Read the model definition and answer for the solid it produces. Units are mm, in the model's axes. Face numbers are marked on the shaded views. A direction names the side the tool comes from. Coordinates: 2 decimals unless noted, no trailing zeros. Write each loop counter-clockwise with the first axis right and the second up, starting at its lowest first coordinate (ties: lowest second). Pieces come first, ordered by that corner, then holes. Notation, with made-up numbers: (10.25, 60) -> (68.25, 60) arc R23 ccw to (68.25, 97) -> close; hole circle Ø11 at (-22, -4). An arc over 180 degrees is marked (long way). Answer as a JSON object with one key per item and string values. Group by question number.
(1) Find section C-C (z = -11). Give the vertices of the cut face in (x, y).
(2) Find section D-D (y = 47). Count the separate pieces of the cut face and the enclosed holes in it, then the cut area to 3 significant figures.
(3) Find section B-B (y = 22). Give the vertices of the cut face in (x, z) (3 decimals).
(4) Which of the six approach directions +Z, -Z, +X, -X, +Y, -Y give full straight-line access (tool end or side, diameter ignored) to the marked faces 4, 5, 6 and 7?
(5) Flat-ended cylindrical pins translate along their axes: P1, Ø1, axis at x = 3, y = 44, coming from the -Z side; P2, Ø1.6, axis at y = 22, z = 15.5, coming from the +X side; P3, Ø1.5, axis at x = 11.5, y = 43.5, coming from the +Z side; P4, Ø2.5, axis at x = 0, y = 47, coming from the -Z side. Find the tip coordinate at first contact, or state that the pin passes through.
(6) Find section A-A (y = 32). Give the vertices of the cut face in (x, z) (3 decimals).
(7) Straight lines are drawn through the part: L1, parallel to Z at x = -5, y = 45.5 (3 decimals); L2, parallel to Z at x = 0.5, y = 24.5 (3 decimals); L3, parallel to Z at x = -9, y = 54. For each, find the intervals that lie inside material, in ascending order.
(8) For a pull along X with two mould halves and no side action, classify the marked faces 1, 2 and 3 as +X half, -X half, draft (parallel to the pull), parting line (faces both ways), or undercut.
from build123d import *

# Parameters (mm, degrees)
SKETCH1_R           = 18
SKETCH1_R_2         = 2
SKETCH1_W           = 10.25
SKETCH1_H           = 10.25
BOSS_EXTRUDE1_DEPTH = 57
CUT_EXTRUDE1_START  = -7
CUT_EXTRUDE1_DEPTH  = 7
SKETCH4_W           = 9.35
SKETCH4_H           = 9.35
CUT_EXTRUDE3_DEPTH  = 20.4
CUT_EXTRUDE4_START  = -40
CUT_EXTRUDE4_DEPTH  = 40
SKETCH6_R           = 1.5
CUT_EXTRUDE5_DEPTH  = 70.267597042
SKETCH7_R           = 3
CUT_EXTRUDE6_DEPTH  = 3
CUT_EXTRUDE7_DEPTH  = 4
CHAMFER1_SIZE       = 1
CHAMFER1_SIZE_2     = 2.747477419
CUT_EXTRUDE8_DEPTH  = 63.42595614
SKETCH12_R          = 1.4
CUT_EXTRUDE10_DEPTH = 20


with BuildPart() as part:
    # Sketch1 → Boss-Extrude1 (new body)
    with BuildSketch(Plane(origin=(0, 0, 0), x_dir=(1, 0, 0), z_dir=(0, 1, 0))):
        with Locations(Location((0, 0, 0), (0, 0, 90))):
            Circle(SKETCH1_R)
        with Locations(Location((-12, 0, 0), (0, 0, 90))):
            Circle(SKETCH1_R_2, mode=Mode.SUBTRACT)
        Rectangle(SKETCH1_W, SKETCH1_H, mode=Mode.SUBTRACT)
    extrude(amount=BOSS_EXTRUDE1_DEPTH)

    # Sketch2 → Cut-Extrude1 (cut)
    with BuildSketch(Plane(origin=(0, 57, 0), x_dir=(1, 0, 0), z_dir=(0, 1, 0)).offset(CUT_EXTRUDE1_START)):
        with BuildLine():
            Line((-10.8, 5), (-17.291616466, 5))
            ThreePointArc((-17.291616466, 5), (-18, 0), (-17.291616466, -5))
            Line((-17.291616466, -5), (-10.8, -5))
            ThreePointArc((-10.8, -5), (-5.8, 0), (-10.8, 5))
        make_face()
    extrude(amount=CUT_EXTRUDE1_DEPTH, mode=Mode.SUBTRACT)

    # Sketch4 → Cut-Extrude3 (cut)
    with BuildSketch(Plane(origin=(0, 0, 0), x_dir=(-1, 0, 0), z_dir=(0, -1, 0))):
        with Locations((11.135393506, 0.872889968)):
            Rectangle(SKETCH4_W, SKETCH4_H)
    extrude(amount=-CUT_EXTRUDE3_DEPTH, mode=Mode.SUBTRACT)

    # Sketch5 → Cut-Extrude4 (cut)
    with BuildSketch(Plane(origin=(0, 57, 0), x_dir=(1, 0, 0), z_dir=(0, 1, 0)).offset(CUT_EXTRUDE4_START)):
        with BuildLine():
            Line((5.916079783, 17), (-5.916079783, 17))
            ThreePointArc((-5.916079783, 17), (0, 18), (5.916079783, 17))
        make_face()
        with BuildLine():
            Line((5.916079783, -17), (-5.916079783, -17))
            ThreePointArc((-5.916079783, -17), (0, -18), (5.916079783, -17))
        make_face()
    extrude(amount=CUT_EXTRUDE4_DEPTH, mode=Mode.SUBTRACT)

    # Sketch6 → Cut-Extrude5 (cut, through all)
    with BuildSketch(Plane(origin=(0, 0, -17), x_dir=(-1, 0, 0), z_dir=(0, 0, -1))):
        with Locations((0, 47)):
            Circle(SKETCH6_R)
        with Locations((0, 22)):
            Circle(SKETCH6_R)
    extrude(amount=-CUT_EXTRUDE5_DEPTH, mode=Mode.SUBTRACT)

    # Sketch7 → Cut-Extrude6 (cut)
    with BuildSketch(Plane(origin=(0, 0, -17), x_dir=(-1, 0, 0), z_dir=(0, 0, -1))):
        with Locations((0, 47)):
            Circle(SKETCH7_R)
        with Locations((0, 22)):
            Circle(SKETCH7_R)
    extrude(amount=-CUT_EXTRUDE6_DEPTH, mode=Mode.SUBTRACT)

    # Sketch8 → Cut-Extrude7 (cut)
    with BuildSketch(Plane.XY.offset(17)):
        Polygon((0, 43.8), (2.771281292, 45.4), (2.771281292, 48.6), (0, 50.2), (-2.771281292, 48.6), (-2.771281292, 45.4), align=None)
        Polygon((0, 18.8), (2.771281292, 20.4), (2.771281292, 23.6), (0, 25.2), (-2.771281292, 23.6), (-2.771281292, 20.4), align=None)
    extrude(amount=-CUT_EXTRUDE7_DEPTH, mode=Mode.SUBTRACT)

    # Chamfer1
    # the kernel refuses this chamfer: 2.747477419, 1 mm, written as the material it takes off along each edge
    with BuildSketch(Plane(origin=(-5.125, 57, -5.125), x_dir=(0, 0.09904090225204956, -0.9950833631817488), z_dir=(1, 0, 0)), Plane(origin=(-5.125, 57, 5.125), x_dir=(-0.9950833631817488, 0.09904090225204956, 0), z_dir=(0, 0, -1)), Plane(origin=(5.125, 57, 5.125), x_dir=(0, 0.09904090225204956, 0.9950833631817488), z_dir=(-1, 0, 0)), Plane(origin=(5.125, 57, -5.125), x_dir=(0.9950833631817488, 0.09904090225204956, 0), z_dir=(0, 0, 1))) as chamfer1_piece_1:
        Polygon((CHAMFER1_SIZE * 0.995083363182, -CHAMFER1_SIZE * 0.099040902252), (-CHAMFER1_SIZE_2 * 0.0990409022684, -CHAMFER1_SIZE_2 * 0.995083363346), (0, 0), align=None)
    extrude(amount=10.25, mode=Mode.SUBTRACT)
    with BuildSketch(Plane(origin=(-5.125, 57, 5.125), x_dir=(-0.9950833631817488, 0.09904090225204956, 0), z_dir=(0, 0, -1))) as chamfer1_piece_2a_section:
        Polygon((CHAMFER1_SIZE * 0.995083363182, -CHAMFER1_SIZE * 0.099040902252), (-CHAMFER1_SIZE_2 * 0.0990409022684, -CHAMFER1_SIZE_2 * 0.995083363346), (0, 0), align=None)
    chamfer1_piece_2a = extrude(amount=17.377491449, mode=Mode.PRIVATE)
    chamfer1_piece_2a = split(chamfer1_piece_2a, bisect_by=Plane(origin=(-5.432505006, 56.059901151, -5.125), z_dir=(0, 0, -1)), keep=Keep.TOP, mode=Mode.PRIVATE)
    with BuildSketch(Plane(origin=(-12.252491449, 57, -5.125), x_dir=(0, 0.09904090225204956, -0.9950833631817488), z_dir=(1, 0, 0))) as chamfer1_piece_2b_section:
        Polygon((CHAMFER1_SIZE * 0.995083363182, -CHAMFER1_SIZE * 0.099040902252), (-CHAMFER1_SIZE_2 * 0.0990409022684, -CHAMFER1_SIZE_2 * 0.995083363346), (0, 0), align=None)
    chamfer1_piece_2b = extrude(amount=17.377491449, mode=Mode.PRIVATE)
    chamfer1_piece_2b = split(chamfer1_piece_2b, bisect_by=Plane(origin=(-5.125, 56.059901151, -5.432505006), z_dir=(-1, 0, 0)), keep=Keep.TOP, mode=Mode.PRIVATE)
    chamfer1_piece_2 = chamfer1_piece_2a & chamfer1_piece_2b
    add(chamfer1_piece_2, mode=Mode.SUBTRACT)
    with BuildSketch(Plane(origin=(5.125, 57, -12.252491449), x_dir=(0.9950833631817488, 0.09904090225204956, 0), z_dir=(0, 0, 1))) as chamfer1_piece_3a_section:
        Polygon((CHAMFER1_SIZE * 0.995083363182, -CHAMFER1_SIZE * 0.099040902252), (-CHAMFER1_SIZE_2 * 0.0990409022684, -CHAMFER1_SIZE_2 * 0.995083363346), (0, 0), align=None)
    chamfer1_piece_3a = extrude(amount=17.377491449, mode=Mode.PRIVATE)
    chamfer1_piece_3a = split(chamfer1_piece_3a, bisect_by=Plane(origin=(5.432505006, 56.059901151, -5.125), z_dir=(0, 0, -1)), keep=Keep.TOP, mode=Mode.PRIVATE)
    with BuildSketch(Plane(origin=(-5.125, 57, -5.125), x_dir=(0, 0.09904090225204956, -0.9950833631817488), z_dir=(1, 0, 0))) as chamfer1_piece_3b_section:
        Polygon((CHAMFER1_SIZE * 0.995083363182, -CHAMFER1_SIZE * 0.099040902252), (-CHAMFER1_SIZE_2 * 0.0990409022684, -CHAMFER1_SIZE_2 * 0.995083363346), (0, 0), align=None)
    chamfer1_piece_3b = extrude(amount=17.377491449, mode=Mode.PRIVATE)
    chamfer1_piece_3b = split(chamfer1_piece_3b, bisect_by=Plane(origin=(5.125, 56.059901151, -5.432505006), z_dir=(1, 0, 0)), keep=Keep.TOP, mode=Mode.PRIVATE)
    chamfer1_piece_3 = chamfer1_piece_3a & chamfer1_piece_3b
    add(chamfer1_piece_3, mode=Mode.SUBTRACT)
    with BuildSketch(Plane(origin=(5.125, 57, 5.125), x_dir=(0, 0.09904090225204956, 0.9950833631817488), z_dir=(-1, 0, 0))) as chamfer1_piece_4a_section:
        Polygon((CHAMFER1_SIZE * 0.995083363182, -CHAMFER1_SIZE * 0.099040902252), (-CHAMFER1_SIZE_2 * 0.0990409022684, -CHAMFER1_SIZE_2 * 0.995083363346), (0, 0), align=None)
    chamfer1_piece_4a = extrude(amount=17.377491449, mode=Mode.PRIVATE)
    chamfer1_piece_4a = split(chamfer1_piece_4a, bisect_by=Plane(origin=(-5.125, 56.059901151, 5.432505006), z_dir=(-1, 0, 0)), keep=Keep.TOP, mode=Mode.PRIVATE)
    with BuildSketch(Plane(origin=(-5.125, 57, 12.252491449), x_dir=(-0.9950833631817488, 0.09904090225204956, 0), z_dir=(0, 0, -1))) as chamfer1_piece_4b_section:
        Polygon((CHAMFER1_SIZE * 0.995083363182, -CHAMFER1_SIZE * 0.099040902252), (-CHAMFER1_SIZE_2 * 0.0990409022684, -CHAMFER1_SIZE_2 * 0.995083363346), (0, 0), align=None)
    chamfer1_piece_4b = extrude(amount=17.377491449, mode=Mode.PRIVATE)
    chamfer1_piece_4b = split(chamfer1_piece_4b, bisect_by=Plane(origin=(-5.432505006, 56.059901151, 5.125), z_dir=(0, 0, 1)), keep=Keep.TOP, mode=Mode.PRIVATE)
    chamfer1_piece_4 = chamfer1_piece_4a & chamfer1_piece_4b
    add(chamfer1_piece_4, mode=Mode.SUBTRACT)
    with BuildSketch(Plane(origin=(12.252491449, 57, 5.125), x_dir=(0, 0.09904090225204956, 0.9950833631817488), z_dir=(-1, 0, 0))) as chamfer1_piece_5a_section:
        Polygon((CHAMFER1_SIZE * 0.995083363182, -CHAMFER1_SIZE * 0.099040902252), (-CHAMFER1_SIZE_2 * 0.0990409022684, -CHAMFER1_SIZE_2 * 0.995083363346), (0, 0), align=None)
    chamfer1_piece_5a = extrude(amount=17.377491449, mode=Mode.PRIVATE)
    chamfer1_piece_5a = split(chamfer1_piece_5a, bisect_by=Plane(origin=(5.125, 56.059901151, 5.432505006), z_dir=(1, 0, 0)), keep=Keep.TOP, mode=Mode.PRIVATE)
    with BuildSketch(Plane(origin=(5.125, 57, -5.125), x_dir=(0.9950833631817488, 0.09904090225204956, 0), z_dir=(0, 0, 1))) as chamfer1_piece_5b_section:
        Polygon((CHAMFER1_SIZE * 0.995083363182, -CHAMFER1_SIZE * 0.099040902252), (-CHAMFER1_SIZE_2 * 0.0990409022684, -CHAMFER1_SIZE_2 * 0.995083363346), (0, 0), align=None)
    chamfer1_piece_5b = extrude(amount=17.377491449, mode=Mode.PRIVATE)
    chamfer1_piece_5b = split(chamfer1_piece_5b, bisect_by=Plane(origin=(5.432505006, 56.059901151, 5.125), z_dir=(0, 0, 1)), keep=Keep.TOP, mode=Mode.PRIVATE)
    chamfer1_piece_5 = chamfer1_piece_5a & chamfer1_piece_5b
    add(chamfer1_piece_5, mode=Mode.SUBTRACT)

    # Sketch9 → Cut-Extrude8 (cut, through all)
    with BuildSketch(Plane.XZ):
        with BuildLine():
            Line((-7.454203172, -7.297889968), (-15.454203172, -7.297889968))
            ThreePointArc((-15.454203172, -7.297889968), (-13.761984914, -9.955415688), (-11.632322635, -12.277178848))
            Line((-11.632322635, -12.277178848), (-7.454203172, -7.297889968))
        make_face()
    extrude(amount=-CUT_EXTRUDE8_DEPTH, mode=Mode.SUBTRACT)

    # Sketch12 → Cut-Extrude10 (cut)
    with BuildSketch(Plane(origin=(0, 57, 0), x_dir=(1, 0, 0), z_dir=(0, 1, 0))):
        with Locations(Location((10, 0, 0), (0, 0, 270))):
            Circle(SKETCH12_R)
        with Locations(Location((-9.192388155, -9.192388155, 0), (0, 0, 270))):
            Circle(SKETCH12_R)
    extrude(amount=-CUT_EXTRUDE10_DEPTH, mode=Mode.SUBTRACT)


solid = part.part
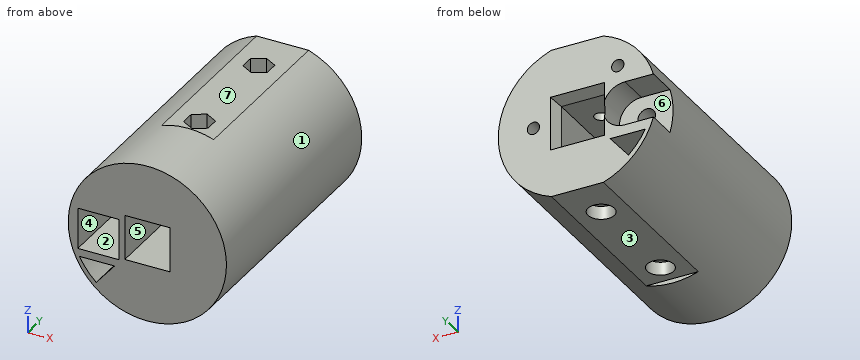
Results below:
{
 "1": {"outline": "(-14.25, 0) -> (-12.9, 0) -> (-12.9, 57) -> (-14.25, 57) -> close; (-10.56, 0) -> (14.25, 0) -> (14.25, 57) -> (-10.56, 57) -> close; hole circle Ø3 at (0, 22); hole circle Ø3 at (0, 47)"},
 "2": {"separate pieces": "2", "enclosed holes": "4", "area": "761 mm2"},
 "3": {"outline": "(-5.916, -17) -> (-3, -17) -> (-3, -14) -> (-1.5, -14) -> (-1.5, -5.125) -> (-5.125, -5.125) -> (-5.125, 5.125) -> (-1.5, 5.125) -> (-1.5, 13) -> (-2.771, 13) -> (-2.771, 17) -> (-5.916, 17) arc R18 ccw to start; (1.5, -14) -> (3, -14) -> (3, -17) -> (5.916, -17) arc R18 ccw to (5.916, 17) -> (2.771, 17) -> (2.771, 13) -> (1.5, 13) -> (1.5, 5.125) -> (5.125, 5.125) -> (5.125, -5.125) -> (1.5, -5.125) -> close; hole (-15.454, -7.298) arc R18 ccw to (-11.632, -12.277) -> (-7.454, -7.298) -> close; hole circle Ø4 at (-12, 0)"},
 "4": {"face 4": "-Y", "face 5": "+Y, -Y", "face 6": "-X, +Y", "face 7": "+Z, +X, -X, +Y"},
 "5": {"P1": "stops at z = -17", "P2": "stops at x = 10.39", "P3": "stops at z = 14.44", "P4": "passes through"},
 "6": {"outline": "(-5.916, -17) -> (5.916, -17) arc R18 ccw to (5.916, 17) -> (-5.916, 17) arc R18 ccw to start; hole (-15.454, -7.298) arc R18 ccw to (-11.632, -12.277) -> (-7.454, -7.298) -> close; hole circle Ø4 at (-12, 0); hole (-5.125, -5.125) -> (5.125, -5.125) -> (5.125, 5.125) -> (-5.125, 5.125) -> close"},
 "7": {"L1": "z = -17 to -5.125, 5.125 to 17", "L2": "z = -14 to -5.125, 5.125 to 13", "L3": "z = -15.59 to -9.14, -7.3 to -4.66, 4.66 to 7.81, 10.58 to 15.59"},
 "8": {"face 1": "parting line", "face 2": "undercut", "face 3": "draft"}
}
